```python
from build123d import *

# Parameters (mm, degrees)
SKETCH1_R                       = 2.25
BOSS_EXTRUDE1_DEPTH             = 14
SKETCH2_W                       = 18
SKETCH2_H                       = 9.25
CUT_EXTRUDE1_DEPTH              = 24.849790355
BOSS_EXTRUDE2_DEPTH             = 2.6
BOSS_EXTRUDE2_DEPTH_BACK        = 2.6
SKETCH4_R                       = 2.25
BOSS_EXTRUDE3_DEPTH             = 28
SKETCH7_W                       = 4.5
SKETCH7_H                       = 3
CUT_EXTRUDE2_DEPTH              = 36.082738034
SKETCH9_W                       = 28
SKETCH9_H                       = 2
BOSS_EXTRUDE4_DEPTH             = 48
BOSS_EXTRUDE5_REACH             = 60.209
SKETCH11_W                      = 28
SKETCH11_H                      = 7.313537016
BOSS_EXTRUDE5_DIRECTION_2_REACH = 60.209
SKETCH14_R                      = 2.15
CUT_EXTRUDE6_DEPTH              = 59.208886884
SKETCH15_W                      = 21.813537016
SKETCH15_H                      = 2
BOSS_EXTRUDE6_DEPTH             = 30
CUT_EXTRUDE7_DEPTH              = 2
SKETCH17_W                      = 21.813537016
SKETCH17_H                      = 2
BOSS_EXTRUDE7_DEPTH             = 30
SKETCH19_R                      = 2.15
CUT_EXTRUDE8_DEPTH              = 2
SKETCH20_W                      = 4.44
SKETCH20_H                      = 13.119449404
SKETCH20_W_2                    = 30
SKETCH20_H_2                    = 8.694087612
CUT_EXTRUDE9_DEPTH              = 2


with BuildPart() as part:
    # Sketch1 → Boss-Extrude1 (new, symmetric)
    with BuildSketch(Plane(origin=(0, 0, 0), x_dir=(0, 0, -1), z_dir=(1, 0, 0))):
        with BuildLine():
            Line((2.25, 1.5), (7.25, 1.5))
            Line((7.25, 1.5), (7.25, 8.5))
            Line((7.25, 8.5), (4.25, 8.5))
            ThreePointArc((4.25, 8.5), (0, 12.75), (-4.25, 8.5))
            Line((-4.25, 8.5), (-7.25, 8.5))
            Line((-7.25, 8.5), (-7.25, 1.5))
            Line((-7.25, 1.5), (-2.25, 1.5))
            Line((-2.25, 1.5), (-2.25, -1.5))
            Line((-2.25, -1.5), (2.25, -1.5))
            Line((2.25, -1.5), (2.25, 1.5))
        make_face()
        with Locations((0, 9)):
            Circle(SKETCH1_R, mode=Mode.SUBTRACT)
    extrude(amount=BOSS_EXTRUDE1_DEPTH, both=True)

    # Sketch2 → Cut-Extrude1 (cut, through all)
    with BuildSketch(Plane.XY.offset(7.25)):
        with Locations((0, 8.125)):
            Rectangle(SKETCH2_W, SKETCH2_H)
    extrude(amount=-CUT_EXTRUDE1_DEPTH, mode=Mode.SUBTRACT)

    # Sketch4 → Boss-Extrude2 (add, two sides: drawn at the far end of the back side and taken through both)
    with BuildSketch(Plane(origin=(0, 0, 0), x_dir=(0, 0, -1), z_dir=(1, 0, 0)).offset(-BOSS_EXTRUDE2_DEPTH_BACK)):
        with BuildLine():
            Line((-4.25, 8.5), (-7.25, 8.5))
            Line((-7.25, 8.5), (-7.25, 3.5))
            Line((-7.25, 3.5), (7.25, 3.5))
            Line((7.25, 3.5), (7.25, 8.5))
            Line((7.25, 8.5), (4.25, 8.5))
            ThreePointArc((4.25, 8.5), (0, 12.75), (-4.25, 8.5))
        make_face()
        with Locations(Location((0, 9, 0), (0, 0, 180))):
            Circle(SKETCH4_R, mode=Mode.SUBTRACT)
    extrude(amount=BOSS_EXTRUDE2_DEPTH + BOSS_EXTRUDE2_DEPTH_BACK)

    # Sketch6 → Boss-Extrude3 (add, through all)
    with BuildSketch(Plane.ZY.offset(14)):
        Polygon((7.25, 8.5), (14.563537016, 15.319983601), (14.563537016, 8.319983601), (7.25, 1.5), align=None)
    extrude(amount=-BOSS_EXTRUDE3_DEPTH)

    # Sketch7 → Cut-Extrude2 (cut, through all)
    with BuildSketch(Plane.ZY.offset(14)):
        Rectangle(SKETCH7_W, SKETCH7_H)
    extrude(amount=-CUT_EXTRUDE2_DEPTH, mode=Mode.SUBTRACT)

    # Sketch9 → Boss-Extrude4 (add)
    with BuildSketch(Plane(origin=(0, 0, -7.25), x_dir=(-1, 0, 0), z_dir=(0, 0, -1))):
        with Locations((0, 2.5)):
            Rectangle(SKETCH9_W, SKETCH9_H)
    extrude(amount=BOSS_EXTRUDE4_DEPTH)

    # Boss-Extrude5: up to this face of the body (flat: up to its plane)
    boss_extrude5_end = Plane(part.part.faces().sort_by_distance((0, 1.5, -24))[0])
    # Sketch11 → Boss-Extrude5 (add, up to the picked face)
    with BuildSketch(Plane(origin=(0, 3.5, 0), x_dir=(1, 0, 0), z_dir=(0, 1, 0)), mode=Mode.PRIVATE) as boss_extrude5_sk1:
        with Locations((0, -10.906768508)):
            Rectangle(SKETCH11_W, SKETCH11_H)
    boss_extrude5_tool1 = split(extrude(boss_extrude5_sk1.sketch, amount=-BOSS_EXTRUDE5_REACH, mode=Mode.PRIVATE), bisect_by=boss_extrude5_end, keep=Keep.BOTH, mode=Mode.PRIVATE)
    add(boss_extrude5_tool1.solids().sort_by(Axis((0, 3.5, 10.906769), (0, -1, 0)))[0])

    # Boss-Extrude5 direction 2: up to this face of the body (flat: up to its plane)
    boss_extrude5_direction_2_end = Plane(part.part.faces().sort_by_distance((0, 4.9099918, 10.906768508))[0])
    # Sketch11 → Boss-Extrude5 direction 2 (add, up to the picked face)
    with BuildSketch(Plane(origin=(0, 3.5, 0), x_dir=(1, 0, 0), z_dir=(0, 1, 0)), mode=Mode.PRIVATE) as boss_extrude5_direction_2_sk1:
        with Locations((0, -10.906768508)):
            Rectangle(SKETCH11_W, SKETCH11_H)
    boss_extrude5_direction_2_tool1 = split(extrude(boss_extrude5_direction_2_sk1.sketch, amount=BOSS_EXTRUDE5_DIRECTION_2_REACH, mode=Mode.PRIVATE), bisect_by=boss_extrude5_direction_2_end, keep=Keep.BOTH, mode=Mode.PRIVATE)
    add(boss_extrude5_direction_2_tool1.solids().sort_by(Axis((0, 3.5, 10.906769), (0, 1, 0)))[0])

    # Sketch14 → Cut-Extrude6 (cut, through all)
    with BuildSketch(Plane(origin=(0, 3.5, 0), x_dir=(1, 0, 0), z_dir=(0, 1, 0))):
        with Locations(Location((11, 51, 0), (0, 0, 270))):
            Circle(SKETCH14_R)
        with Locations(Location((11, 29, 0), (0, 0, 270))):
            Circle(SKETCH14_R)
        with Locations(Location((-11, 29, 0), (0, 0, 270))):
            Circle(SKETCH14_R)
        with Locations(Location((-11, 51, 0), (0, 0, 270))):
            Circle(SKETCH14_R)
    extrude(amount=-CUT_EXTRUDE6_DEPTH, mode=Mode.SUBTRACT)

    # Sketch15 → Boss-Extrude6 (add)
    with BuildSketch(Plane(origin=(14, 0, 0), x_dir=(0, 0, -1), z_dir=(1, 0, 0))):
        with Locations((-3.656768508, 2.5)):
            Rectangle(SKETCH15_W, SKETCH15_H)
    extrude(amount=BOSS_EXTRUDE6_DEPTH)

    # Sketch16 → Cut-Extrude7 (cut)
    with BuildSketch(Plane(origin=(0, 3.5, 0), x_dir=(1, 0, 0), z_dir=(0, 1, 0))):
        with BuildLine():
            ThreePointArc((33, -5.854087612), (32.430271679, -5.930947569), (31.901277584, -6.156032133))
            Line((31.901277584, -6.156032133), (33, -8.004087612))
            Line((33, -8.004087612), (33, -5.854087612))
        make_face()
        with BuildLine():
            Line((33, -8.004087612), (31.901277584, -6.156032133))
            ThreePointArc((31.901277584, -6.156032133), (31.936927376, -9.872877755), (35.15, -8.004087612))
            ThreePointArc((35.15, -8.004087612), (34.52027958, -6.483808032), (33, -5.854087612))
            Line((33, -5.854087612), (33, -8.004087612))
        make_face()
    extrude(amount=-CUT_EXTRUDE7_DEPTH, mode=Mode.SUBTRACT)

    # Sketch17 → Boss-Extrude7 (add)
    with BuildSketch(Plane.ZY.offset(14)):
        with Locations((3.656768508, 2.5)):
            Rectangle(SKETCH17_W, SKETCH17_H)
    extrude(amount=BOSS_EXTRUDE7_DEPTH)

    # Sketch19 → Cut-Extrude8 (cut)
    with BuildSketch(Plane(origin=(0, 3.5, 0), x_dir=(1, 0, 0), z_dir=(0, 1, 0))):
        with Locations(Location((-33, -8, 0), (0, 0, 270))):
            Circle(SKETCH19_R)
    extrude(amount=-CUT_EXTRUDE8_DEPTH, mode=Mode.SUBTRACT)

    # Sketch20 → Cut-Extrude9 (cut)
    with BuildSketch(Plane(origin=(0, 3.5, 0), x_dir=(1, 0, 0), z_dir=(0, 1, 0))):
        Polygon((44, 7.25), (14, 7.25), (14, -1.444087612), (39.56, -1.444087612), (44, -1.444087612), align=None)
        with Locations((41.78, -8.003812314)):
            Rectangle(SKETCH20_W, SKETCH20_H)
        with Locations((-29, 2.902956194)):
            Rectangle(SKETCH20_W_2, SKETCH20_H_2)
        with Locations((-41.78, -8.003812314)):
            Rectangle(SKETCH20_W, SKETCH20_H)
    extrude(amount=-CUT_EXTRUDE9_DEPTH, mode=Mode.SUBTRACT)


solid = part.part
```
The listing builds one solid part. Answer for the finished solid, in the listing's coordinates (mm). A direction names the side the tool comes from. Coordinates: 2 decimals unless noted, no trailing zeros. Loops run counter-clockwise (first coordinate to the right, second up) from the corner with the lowest first, then second, coordinate; pieces in that order, holes last. Notation, with made-up numbers: (29, 8) -> (50, 8) arc R18 ccw to (50, 41) -> close; hole circle Ø8 at (75, -38.5). An arc over 180 degrees is marked (long way). Return JSON: item names as keys, results as strings. Group by question number.
(1) Find the intervals of material crossed by probe 1 along X at (y, z) = (2.4, 8); probe 2 along X at (y, z) = (2.8, -29); probe 3 along Y at (x, z) = (-12.6, 0), in increasing order. Write a range as from..to.
(2) A cutting plane is placed at B-B on x = -11. Write down the section's boundary in (y, z).
(3) A cutting plane is placed at A-A on x = -33. Write down the section's boundary in (y, z), and give its area (3 significant figures).
(4) Which of the six approach directions +Z, -Z, +X, -X, +Y, -Y give full straight-line access (tool end or side, diameter ignored) to faces 4 (the flat face through (12, 8.5, 6)), 5 (the flat face through (-27, 3.5, 8)), 6 (the flat face through (0, 3.5, -24))?
(5) A cutting plane is placed at D-D on z = 0. Write down the section's boundary in (x, y).
(6) Determine the mould class of faces 1 (the flat face through (14, 3, -7)), 2 (the flat face through (12, 6, -7.25)), 3 (the cylindrical face through (-11.46, 12.75, -0.09)) for opening direction Z: released by +Z, released by -Z, zero draft, split by the parting line, or undercut.
(7) A cutting plane is placed at C-C on z = -28.5. Write down the section's boundary in (x, y).
(8) Given pin 1 Ø0.9 at (x, z) = (0.5, 6.5) entering from +Y; pin 2 Ø10.5 at (x, z) = (-27, 7) entering from +Y; pin 3 Ø1.6 at (x, y) = (31.5, 2) entering from -Z, each flat-ended and moving along its own axis, determine where each tip first touches the part or whether it passes through.
The answers:
{
 "1": {"probe 1": "x = -39.56..-35.15, -30.85..30.85, 35.15..39.56", "probe 2": "x = -14..-13.15, -8.85..8.85, 13.15..14", "probe 3": "y = 1.5..6.75, 11.25..12.75"},
 "2": {"outline": "(1.5, -55.25) -> (3.5, -55.25) -> (3.5, -53.15) -> (1.5, -53.15) -> close; (1.5, -48.85) -> (3.5, -48.85) -> (3.5, -31.15) -> (1.5, -31.15) -> close; (1.5, -26.85) -> (3.5, -26.85) -> (3.5, -7.25) -> (8.5, -7.25) -> (8.5, -4.25) arc R4.25 ccw to (8.5, 4.25) -> (8.5, 7.25) -> (15.32, 14.56) -> (1.5, 14.56) -> close; hole circle Ø4.5 at (9, 0)"},
 "3": {"outline": "(1.5, 1.44) -> (3.5, 1.44) -> (3.5, 5.85) -> (1.5, 5.85) -> close; (1.5, 10.15) -> (3.5, 10.15) -> (3.5, 14.56) -> (1.5, 14.56) -> close", "area": "17.6 mm^2"},
 "4": {"face 4": "+X, -X, +Y", "face 5": "+Z, -Z, -X, +Y", "face 6": "-Z, +Y"},
 "5": {"outline": "(-14, 1.5) -> (14, 1.5) -> (14, 6.75) -> (9, 6.75) -> (9, 3.5) -> (2.6, 3.5) -> (2.6, 6.75) -> (-2.6, 6.75) -> (-2.6, 3.5) -> (-9, 3.5) -> (-9, 6.75) -> (-14, 6.75) -> close; (-14, 11.25) -> (-9, 11.25) -> (-9, 12.75) -> (-14, 12.75) -> close; (-2.6, 11.25) -> (2.6, 11.25) -> (2.6, 12.75) -> (-2.6, 12.75) -> close; (9, 11.25) -> (14, 11.25) -> (14, 12.75) -> (9, 12.75) -> close"},
 "6": {"face 1": "zero draft", "face 2": "released by -Z", "face 3": "undercut"},
 "7": {"outline": "(-14, 1.5) -> (-13.09, 1.5) -> (-13.09, 3.5) -> (-14, 3.5) -> close; (-8.91, 1.5) -> (8.91, 1.5) -> (8.91, 3.5) -> (-8.91, 3.5) -> close; (13.09, 1.5) -> (14, 1.5) -> (14, 3.5) -> (13.09, 3.5) -> close"},
 "8": {"pin 1": "stops at y = 8.5", "pin 2": "stops at y = 3.5", "pin 3": "stops at z = 1.44"}
}
